Can you work these out from the model? Positions are in its coordinate system, mm. A direction names the side the tool comes from. Coordinates: 2 decimals unless noted, no trailing zeros. Loops run counter-clockwise (first coordinate to the right, second up) from the corner with the lowest first, then second, coordinate; pieces in that order, holes last.
```python
from build123d import *

# Parameters (mm, degrees)
PAD_DEPTH    = 400
POCKET_DEPTH = 350
FILLET_R     = 100


with BuildPart() as part:
    # Sketch → Pad (new body)
    with BuildSketch(Plane.XZ):
        with BuildLine():
            Line((100, 0), (1400, 0))
            ThreePointArc((1400, 0), (1470.710678, 29.289322), (1500, 100))
            Line((1500, 100), (1500, 650))
            ThreePointArc((1500, 650), (1470.710678, 720.710678), (1400, 750))
            Line((1400, 750), (100, 750))
            ThreePointArc((100, 750), (29.289322, 720.710678), (0, 650))
            Line((0, 650), (0, 100))
            ThreePointArc((0, 100), (29.289322, 29.289322), (100, 0))
        make_face()
    extrude(amount=PAD_DEPTH)

    # Sketch001 (on Face9 of Pad) → Pocket (cut)
    with BuildSketch(Plane(origin=(0, 0, 0), x_dir=(1, 0, 0), z_dir=(0, 1, 0))):
        with BuildLine():
            Line((80, -130), (80, -629.552775))
            ThreePointArc((80, -629.552775), (94.644661, -664.908114), (130, -679.552775))
            Line((130, -679.552775), (1369.052368, -679.552775))
            ThreePointArc((1369.052368, -679.552775), (1404.407707, -664.908114), (1419.052368, -629.552775))
            Line((1419.052368, -629.552775), (1419.052368, -130))
            ThreePointArc((1419.052368, -130), (1404.407707, -94.644661), (1369.052368, -80))
            Line((1369.052368, -80), (130, -80))
            ThreePointArc((130, -80), (94.644661, -94.644661), (80, -130))
        make_face()
    extrude(amount=-POCKET_DEPTH, mode=Mode.SUBTRACT)

    # Fillet
    fillet_edges = [part.edges().sort_by_distance(p)[0] for p in [
        (80, -350, 379.776388),
        (94.644661, -350, 664.908114),
        (749.526184, -350, 679.552775),
        (1404.407707, -350, 664.908114),
        (1419.052368, -350, 379.776388),
        (1404.407707, -350, 94.644661),
        (749.526184, -350, 80),
        (94.644661, -350, 94.644661),
    ]]
    fillet(fillet_edges, radius=FILLET_R)


solid = part.part
```
(1) I'm going to push flat-ended pins straight in: pin 1 (6 mm diameter, centred on x = 618.5, z = 538, fed in from +Y); pin 2 (3 mm diameter, centred on x = 806, y = -324.5, fed in from -Z). Where does each tip first touch, or does it pass through?
Check values:
pin 1: stops at y = -350
pin 2: stops at z = 0
(2) I want a section at B-B on x = 320.5. Write out the boundary of the cut face in (y, z).
Check values:
outline: (-400, 0) - (0, 0) - (0, 80) - (-250, 80) arc R100 cw to (-350, 180) - (-350, 579.55) arc R100 cw to (-250, 679.55) - (0, 679.55) - (0, 750) - (-400, 750) - close
(3) I want a section at A-A on y = -124.5. Write out the boundary of the cut face in (x, z), then the cut area to 3 significant figures.
Check values:
outline: (0, 100) arc R100 ccw to (100, 0) - (1400, 0) arc R100 ccw to (1500, 100) - (1500, 650) arc R100 ccw to (1400, 750) - (100, 750) arc R100 ccw to (0, 650) - close; hole (80, 130) arc R50 ccw to (130, 80) - (1369.05, 80) arc R50 ccw to (1419.05, 130) - (1419.05, 629.55) arc R50 ccw to (1369.05, 679.55) - (130, 679.55) arc R50 ccw to (80, 629.55) - close
area: 316,000 mm2
(4) If I drill on probe 1 along Z at (x, y) = (471, -61.5); probe 2 along X at (y, z) = (-103.5, 419); probe 3 along Y at (x, z) = (1327, 268), over which ranges is the centre line in solid material (lowest first)?
Check values:
probe 1: z = 0 to 80, 679.55 to 750
probe 2: x = 0 to 80, 1419.05 to 1500
probe 3: y = -400 to -349.68
(5) If we mould it in two halves opening along X, with no side actions, what happens to faces 3 (the cylindrical face through (95.036, -123.25, 94.258)), 4 (the cylindrical face through (1469.929, -197.2, 28.516)), 5 (the flat face through (741, -197, 0))? For each: released by +X, released by -X, zero draft, split by the parting line, or undercut.
Check values:
face 3: undercut
face 4: released by +X
face 5: zero draft
(6) I want a section at C-C on z = 216.5. Write out the boundary of the cut face in (x, y), then the cut area to 3 significant figures.
Check values:
outline: (0, -400) - (1500, -400) - (1500, 0) - (1419.05, 0) - (1419.05, -250) arc R100 cw to (1319.05, -350) - (180, -350) arc R100 cw to (80, -250) - (80, 0) - (0, 0) - close
area: 136,000 mm2
(7) Which directions (+Z, -Z, +X, -X, +Y, -Y) give clear straight access to the entire face, cutting with the end or side of a thin tool? Please do faces 1 (the flat face through (1419.052, -123, 383)), 2 (the flat face through (740, -400, 380)).
Check values:
face 1: +Y
face 2: +Z, -Z, +X, -X, -Y
